Here's how the part is built. I have some questions about the finished solid (model axes, mm). A direction names the side the tool comes from. Round coordinates to 2 decimals unless told otherwise and drop trailing zeros. Write each loop counter-clockwise with the first axis right and the second up, starting at its lowest first coordinate (ties: lowest second). Pieces come first, ordered by that corner, then holes. Notation, with made-up numbers: (45, -33) -> (64, -33) arc R27 cw to (64, -10) -> close; hole circle Ø2 at (-34.75, 58). An arc over 180 degrees is marked (long way). Put each result on its own line as item: value. Start each with the question number.
1. Suppose I cut it at A-A (y = 31.5). Please give me the cut outline in (x, z), then the cut area to 3 significant figures.
2. Suppose I cut it at C-C (x = 40). Please give me the cut outline in (y, z).
3. Which directions (+Z, -Z, +X, -X, +Y, -Y) give clear straight access to the entire face, cutting with the end or side of a thin tool? Please do faces 1 (the face through (100, 55, 10)), 2 (the face through (65, 20, 10)), 3 (the face through (125.07, 4.677, 7.231)), 4 (the face through (30, 35, 10)).
4. For pin 1 (10 mm diameter, centred on y = 66.5, z = 7, fed in from +X); pin 2 (1.5 mm diameter, centred on x = 15.5, z = 12, fed in from +Y); pin 3 (6 mm diameter, centred on y = 40, z = 14.5, fed in from -X), each with a flat end and sliding along its axis, tell me the tip position at first contact or that it passes through.
5. We'd pull the mould along X, two halves only. Please class faces 5 (the face through (130, 10, 10)), 6 (the face through (61, 16, 0)), 7 (the face through (40, 40, 10)), 8 (the face through (80, 55, 10)): +X half, -X half, draft (parallel to the pull), parting line (faces both ways), or undercut.
6. I need wall thicknesses on probe 1 along X at (y, z) = (43, 10); probe 2 along X at (y, z) = (34, 15.75); probe 3 along Y at (x, z) = (73.5, 18.75). Which ranges of each line are inside material? Lowest first, please. Write a range as from..to.
7. Suppose I cut it at B-B (z = 10). Please give me the cut outline in (x, y), then the cut area to 3 significant figures.
8. Suppose I cut it at D-D (y = 10). Please give me the cut outline in (x, z), then the cut area to 3 significant figures.
```python
from build123d import *

# Parameters (mm, degrees)
EXTRUDE1_DEPTH     = 20
SKETCH2_R          = 3
CUT_EXTRUDE2_DEPTH = 10
SKETCH3_OUTSIDE_W  = 53.874
SKETCH3_OUTSIDE_H  = 123.874
SKETCH3_OUTSIDE_R  = 6
CUT_EXTRUDE3_DEPTH = 10


with BuildPart() as part:
    # Sketch1 → Extrude1 (new body)
    with BuildSketch(Plane.XY):
        Polygon((30, 50), (50, 50), (50, 20), (80, 20), (80, 90), (100, 90), (100, 20), (130, 20), (130, 0), (0, 0), (0, 20), (30, 20), align=None)
    extrude(amount=EXTRUDE1_DEPTH)

    # Sketch2 → Cut-Extrude2 (cut)
    with BuildSketch(Plane(origin=(0, 50, 0), x_dir=(-1, 0, 0), z_dir=(0, 1, 0))):
        with Locations(Location((-40, 10, 0), (0, 0, 90))):  # turned: the seam where the file's is
            Circle(SKETCH2_R)
    extrude(amount=-CUT_EXTRUDE2_DEPTH, mode=Mode.SUBTRACT)

    # Sketch3 outside → Cut-Extrude3 (cut)
    with BuildSketch(Plane(origin=(130, 0, 0), x_dir=(0, 0, -1), z_dir=(1, 0, 0))):
        with Locations((-10, 45)):
            Rectangle(SKETCH3_OUTSIDE_W, SKETCH3_OUTSIDE_H)
        with Locations((-10, 10)):
            Circle(SKETCH3_OUTSIDE_R, mode=Mode.SUBTRACT)
    extrude(amount=-CUT_EXTRUDE3_DEPTH, mode=Mode.SUBTRACT)


solid = part.part
```
Verdict:
1. outline: (30, 0) -> (50, 0) -> (50, 20) -> (30, 20) -> close; (80, 0) -> (100, 0) -> (100, 20) -> (80, 20) -> close
1. area: 800 mm^2
2. outline: (0, 0) -> (50, 0) -> (50, 7) -> (40, 7) -> (40, 13) -> (50, 13) -> (50, 20) -> (0, 20) -> close
3. face 1: +Z, -Z, +X, +Y
3. face 2: +Z, -Z, +Y
3. face 3: +X
3. face 4: +Z, -Z, -X, +Y
4. pin 1: stops at x = 100
4. pin 2: stops at y = 20
4. pin 3: stops at x = 30
5. face 5: +X half
5. face 6: draft
5. face 7: undercut
5. face 8: undercut
6. probe 1: x = 30..37, 43..50, 80..100
6. probe 2: x = 30..50, 80..100
6. probe 3: y = 0..20
7. outline: (0, 0) -> (120, 0) -> (120, 4) -> (130, 4) -> (130, 16) -> (120, 16) -> (120, 20) -> (100, 20) -> (100, 90) -> (80, 90) -> (80, 20) -> (50, 20) -> (50, 50) -> (43, 50) -> (43, 40) -> (37, 40) -> (37, 50) -> (30, 50) -> (30, 20) -> (0, 20) -> close
7. area: 4,460 mm^2
8. outline: (0, 0) -> (120, 0) -> (120, 4) -> (130, 4) -> (130, 16) -> (120, 16) -> (120, 20) -> (0, 20) -> close
8. area: 2,520 mm^2
